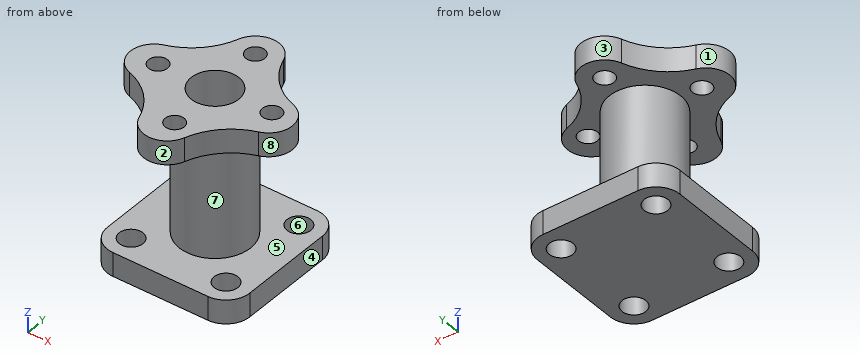
from build123d import *

# Parameters (mm, degrees)
SCHIZZO1_W                   = 120
SCHIZZO1_H                   = 120
ESTRUSIONE_ESTRUSIONE1_DEPTH = 20
SCHIZZO3_R                   = 30
SCHIZZO3_R_2                 = 20
ESTRUSIONE_ESTRUSIONE2_DEPTH = 100
SCHIZZO4_R                   = 20
ESTRUSIONE_ESTRUSIONE3_DEPTH = 20
RACCORDO2_R                  = 20
SCHIZZO8_R                   = 8
TAGLIO_ESTRUSIONE1_DEPTH     = 20
SCHIZZO7_R                   = 10
TAGLIO_ESTRUSIONE2_DEPTH     = 20
RIPETIZIONECIRCOLARE1_COUNT  = 4


with BuildPart() as part:
    # Schizzo1 → Estrusione-Estrusione1 (new body)
    with BuildSketch(Plane.XY):
        Rectangle(SCHIZZO1_W, SCHIZZO1_H)
    extrude(amount=ESTRUSIONE_ESTRUSIONE1_DEPTH)

    # Schizzo3 → Estrusione-Estrusione2 (add)
    with BuildSketch(Plane.XY.offset(20)):
        Circle(SCHIZZO3_R)
        Circle(SCHIZZO3_R_2, mode=Mode.SUBTRACT)
    extrude(amount=ESTRUSIONE_ESTRUSIONE2_DEPTH)

    # Schizzo4 → Estrusione-Estrusione3 (add)
    with BuildSketch(Plane.XY.offset(120)):
        with BuildLine():
            ThreePointArc((-56.205527859, 17.383404463), (-34.252252481, 30.819558816), (-20.816098128, 52.772834194))
            ThreePointArc((-20.816098128, 52.772834194), (-1.788088194, 66.613707799), (17.23992174, 52.772834194))
            ThreePointArc((17.23992174, 52.772834194), (30.676076093, 30.819558816), (52.629351472, 17.383404463))
            ThreePointArc((52.629351472, 17.383404463), (66.470225076, -1.644605471), (52.629351472, -20.672615405))
            ThreePointArc((52.629351472, -20.672615405), (30.676076093, -34.108769758), (17.23992174, -56.062045137))
            ThreePointArc((17.23992174, -56.062045137), (-1.788088194, -69.902918741), (-20.816098128, -56.062045137))
            ThreePointArc((-20.816098128, -56.062045137), (-34.252252481, -34.108769758), (-56.205527859, -20.672615405))
            ThreePointArc((-56.205527859, -20.672615405), (-70.046401464, -1.644605471), (-56.205527859, 17.383404463))
        make_face()
        Circle(SCHIZZO4_R, mode=Mode.SUBTRACT)
    extrude(amount=ESTRUSIONE_ESTRUSIONE3_DEPTH)

    # Raccordo2
    raccordo2_edges = [part.edges().sort_by_distance(p)[0] for p in [
        (-60, 60, 10),
        (60, 60, 10),
        (60, -60, 10),
        (-60, -60, 10),
    ]]
    fillet(raccordo2_edges, radius=RACCORDO2_R)

    # Schizzo8 → Taglio-Estrusione1 (cut)
    with BuildSketch(Plane.XY.offset(140)):
        with Locations((-1.788088194, 46.613707799)):
            Circle(SCHIZZO8_R)
    taglio_estrusione1 = extrude(amount=-TAGLIO_ESTRUSIONE1_DEPTH, mode=Mode.SUBTRACT)

    # Schizzo7 → Taglio-Estrusione2 (cut)
    with BuildSketch(Plane(origin=(0, 0, 0), x_dir=(-1, 0, 0), z_dir=(0, 0, -1))):
        with Locations((-40, 40)):
            Circle(SCHIZZO7_R)
    taglio_estrusione2 = extrude(amount=-TAGLIO_ESTRUSIONE2_DEPTH, mode=Mode.SUBTRACT)

    # RipetizioneCircolare1: Taglio-Estrusione1, Taglio-Estrusione2 ×4 about axis
    ripetizionecircolare1_axis = Axis((0, 0, 0), (0, 0, 1))
    for i in range(1, RIPETIZIONECIRCOLARE1_COUNT):
        add(taglio_estrusione1.rotate(ripetizionecircolare1_axis, i * 360 / RIPETIZIONECIRCOLARE1_COUNT), mode=Mode.SUBTRACT)
        add(taglio_estrusione2.rotate(ripetizionecircolare1_axis, i * 360 / RIPETIZIONECIRCOLARE1_COUNT), mode=Mode.SUBTRACT)


solid = part.part
Model file for the job. Use its own axes, mm. Face numbers are marked on the shaded views. A direction names the side the tool comes from. Give positions to 0.01 mm unless a question says otherwise; leave off trailing zeros. Loops run counter-clockwise (first coordinate to the right, second up) from the corner with the lowest first, then second, coordinate; pieces in that order, holes last. Notation, with made-up numbers: (87, -22) -> (135, -22) arc R17 ccw to (135, -12) -> close; hole circle Ø5 at (-28.5, 6). An arc over 180 degrees is marked (long way). Use a Markdown table: item, result. Add a question column.
(1) Slice it at D-D on y = 42.5. List the corners of the cut face in (x, z).
(2) Drop flat-ended pins along their axis: pin 1 Ø6 at (y, z) = (-14, 11.5) entering from +X; pin 2 Ø12 at (x, y) = (1, -1.5) entering from +Z; pin 3 Ø1 at (y, z) = (-25.5, 47.5) entering from +X. Give the stop position or say it passes through.
(3) Slice it at B-B on x = 0. List the corners of the cut face in (y, z), and give its area (3 significant figures).
(4) Slice it at C-C on x = -35. List the corners of the cut face in (y, z), and give its area (3 significant figures).
(5) Tool access for the marked faces 1, 2, 3, 4 and 5: list every direction of +Z, -Z, +X, -X, +Y, -Y with a clear straight run to the whole face (end or side of a thin tool).
(6) Wall check: line 1 along X through (y, z) = (39.5, 17); line 2 along Z through (x, y) = (-26, -28); line 3 along X through (y, z) = (0.5, 91). Give the ranges that are in metal, low to high.
(7) Slice it at A-A on y = 0. List the corners of the cut face in (x, z), and give its area (3 significant figures).
(8) Mould opens along X. For the marked faces 6, 7 and 8 say: +X half, -X half, draft (parallel to the pull), parting line (faces both ways), or undercut.
Filled sheet:
| question | item | result |
|---|---|---|
| 1 | outline | (-59.84, 0) -> (-49.68, 0) -> (-49.68, 20) -> (-59.84, 20) -> close; (-30.32, 0) -> (30.32, 0) -> (30.32, 20) -> (-30.32, 20) -> close; (-25.35, 120) -> (-8.65, 120) -> (-8.65, 140) -> (-25.35, 140) -> close; (5.07, 120) -> (21.77, 120) -> (21.77, 140) -> (5.07, 140) -> close; (49.68, 0) -> (59.84, 0) -> (59.84, 20) -> (49.68, 20) -> close |
| 2 | pin 1 | x = 60 |
| 2 | pin 2 | z = 20 |
| 2 | pin 3 | x = 16.58 |
| 3 | outline | (-69.82, 120) -> (-54.41, 120) -> (-54.41, 140) -> (-69.82, 140) -> close; (-60, 0) -> (60, 0) -> (60, 20) -> (30, 20) -> (30, 120) -> (38.82, 120) -> (38.82, 140) -> (20, 140) -> (20, 20) -> (-20, 20) -> (-20, 140) -> (-38.82, 140) -> (-38.82, 120) -> (-30, 120) -> (-30, 20) -> (-60, 20) -> close; (54.41, 120) -> (66.53, 120) -> (66.53, 140) -> (54.41, 140) -> close |
| 3 | area | 5,700 mm2 |
| 4 | outline | (-60, 0) -> (-48.66, 0) -> (-48.66, 20) -> (-60, 20) -> close; (-33.38, 120) -> (30.09, 120) -> (30.09, 140) -> (-33.38, 140) -> close; (-31.34, 0) -> (31.34, 0) -> (31.34, 20) -> (-31.34, 20) -> close; (48.66, 0) -> (60, 0) -> (60, 20) -> (48.66, 20) -> close |
| 4 | area | 2,980 mm2 |
| 5 | face 1 | +Z, -X |
| 5 | face 2 | +Z, -Y |
| 5 | face 3 | +Z, +Y |
| 5 | face 4 | -Z, +X, +Y, -Y |
| 5 | face 5 | none |
| 6 | line 1 | -60 to -49.99, -30.01 to 30.01, 49.99 to 60 |
| 6 | line 2 | 0 to 20, 120 to 140 |
| 6 | line 3 | -30 to -19.99, 19.99 to 30 |
| 7 | outline | (-69.98, 120) -> (-54.41, 120) -> (-54.41, 140) -> (-69.98, 140) -> close; (-60, 0) -> (60, 0) -> (60, 20) -> (30, 20) -> (30, 120) -> (38.82, 120) -> (38.82, 140) -> (20, 140) -> (20, 20) -> (-20, 20) -> (-20, 140) -> (-38.82, 140) -> (-38.82, 120) -> (-30, 120) -> (-30, 20) -> (-60, 20) -> close; (54.41, 120) -> (66.4, 120) -> (66.4, 140) -> (54.41, 140) -> close |
| 7 | area | 5,700 mm2 |
| 8 | face 6 | undercut |
| 8 | face 7 | parting line |
| 8 | face 8 | +X half |
